Read the model definition and answer for the solid it produces. Units are mm, in the model's axes. A direction names the side the tool comes from. Coordinates: 2 decimals unless noted, no trailing zeros. Write each loop counter-clockwise with the first axis right and the second up, starting at its lowest first coordinate (ties: lowest second). Pieces come first, ordered by that corner, then holes.
1) The part is cut by section A-A (y = 0). Determine the outline of the cut face in (x, z), then the cut area to 4 significant figures.
2) Each of these flat-tipped pins is pushed along its axis until it touches: pin 1 Ø6 at (x, y) = (0, -12.5) entering from +Z; pin 2 Ø7.5 at (x, y) = (0.5, 0.5) entering from -Z; pin 3 Ø7 at (x, z) = (-3.5, 12.5) entering from -Y. Where does it stop, or does it pass through?
3) The part is cut by section C-C (x = 0). Determine the outline of the cut face in (y, z).
4) The part is cut by section D-D (y = 8.25). Determine the outline of the cut face in (x, z).
5) Determine the mould class of faces 1 (the face through (3.5, 0, 7)), 2 (the face through (0, 6, 9)), 3 (the face through (6, 0, 5)), 4 (the face through (10, 0, 0)) for opening direction Y: +Y half, -Y half, draft (parallel to the pull), parting line (faces both ways), or undercut.
6) Find the intervals of material crossed by line 1 (Y direction, x = 0, z = 12); line 2 (X direction, y = 8, z = -0.5); line 3 (Y direction, x = 0, z = -2), in increasing order.
7) The part is cut by section B-B (z = 0). Determine the outline of the cut face in (x, y), then the cut area to 3 significant figures.
8) Which of the six approach directions +Z, -Z, +X, -X, +Y, -Y give full straight-line access (tool end or side, diameter ignored) to faces 5 (the face through (-2, 2, 8.5)), 6 (the face through (-10, -14, 0)), 7 (the face through (-13.274, -11.268, -3.045))?
from build123d import *

# Parameters (mm, degrees)
BOX002_W               = 12.5
BOX002_H               = 5
BOX002_DEPTH           = 10
CYLINDER003_R          = 2
CYLINDER003_DEPTH      = 30
CYLINDER003_ROLL_ANGLE = -90
CYLINDER_R             = 2
CYLINDER_DEPTH         = 30
CYLINDER007_R          = 10
CYLINDER007_DEPTH      = 40
BOX008_W               = 10
BOX008_H               = 2.5
BOX008_DEPTH           = 10
BOX009_W               = 10
BOX009_H               = 2.5
BOX009_DEPTH           = 10
PAD_DEPTH              = 2.5
BOX010_W               = 7
BOX010_H               = 20
BOX010_DEPTH           = 3.5
CYLINDER001_R          = 10
CYLINDER001_DEPTH      = 10
PAD001_DEPTH           = 40
BOX007_W               = 40
BOX007_H               = 30
BOX007_DEPTH           = 10
BOX_W                  = 40
BOX_H                  = 10
BOX_DEPTH              = 12


with BuildPart() as screw_gap:
    # Box002 → Box002 (new body)
    with BuildSketch(Plane(origin=(-20, -2.5, -5), x_dir=(1, 0, 0), z_dir=(0, 0, 1))):
        with Locations((6.25, 2.5)):
            Rectangle(BOX002_W, BOX002_H)
    extrude(amount=BOX002_DEPTH)


with BuildPart() as screw:
    # Cylinder003 → Cylinder003 (new body)
    with BuildSketch(Plane.XY):
        Circle(CYLINDER003_R)
    extrude(amount=CYLINDER003_DEPTH)


with BuildPart() as screw_1:
    # Cylinder003 roll: moved
    add(screw.part.rotate(Axis((0, 0, 0), (1, 0, 0)), CYLINDER003_ROLL_ANGLE))


with BuildPart() as screw_2:
    # Cylinder003 placement: moved
    add(screw_1.part.moved(Location((-15, -15, 0))))


with BuildPart() as rail_screw:
    # Cylinder → Cylinder (new body)
    with BuildSketch(Plane.XY.offset(-5)):
        Circle(CYLINDER_R)
    extrude(amount=CYLINDER_DEPTH)


with BuildPart() as rail:
    # Cylinder007 → Cylinder007 (new body)
    with BuildSketch(Plane(origin=(20, 0, 25), x_dir=(0, 1, 0), z_dir=(-1, 0, 0))):
        Circle(CYLINDER007_R)
    extrude(amount=CYLINDER007_DEPTH)


with BuildPart() as screw_gap001:
    # Box008 → Box008 (new body)
    with BuildSketch(Plane(origin=(-20, 12.5, -5), x_dir=(1, 0, 0), z_dir=(0, 0, 1))):
        with Locations((5, 1.25)):
            Rectangle(BOX008_W, BOX008_H)
    extrude(amount=BOX008_DEPTH)


with BuildPart() as screw_gap002:
    # Box009 → Box009 (new body)
    with BuildSketch(Plane(origin=(-20, -15, -5), x_dir=(1, 0, 0), z_dir=(0, 0, 1))):
        with Locations((5, 1.25)):
            Rectangle(BOX009_W, BOX009_H)
    extrude(amount=BOX009_DEPTH)


with BuildPart() as body:
    # Sketch → Pad (new body)
    with BuildSketch(Plane.XZ):
        Polygon((0, -4.041452), (3.5, -2.020726), (3.5, 2.020726), (0, 4.041452), (-3.5, 2.020726), (-3.5, -2.020726), align=None)
    extrude(amount=-PAD_DEPTH)


with BuildPart() as body_1:
    # Body placement: moved
    add(body.part.moved(Location((-15, -12.5, 0))))


with BuildPart() as cube:
    # Box010 → Box010 (new body)
    with BuildSketch(Plane(origin=(-3.5, -10, 5), x_dir=(1, 0, 0), z_dir=(0, 0, 1))):
        with Locations((3.5, 10)):
            Rectangle(BOX010_W, BOX010_H)
    extrude(amount=BOX010_DEPTH)


with BuildPart() as negative_fusion:
    # Cylinder001 → Cylinder001 (new body)
    with BuildSketch(Plane.XY.offset(-5)):
        Circle(CYLINDER001_R)
    extrude(amount=CYLINDER001_DEPTH)

    # Fusion: union Screw Gap, Screw, Rail Screw, Rail, Screw Gap001, Screw Gap002, Body, Cube
    add(screw_gap.part)
    add(screw_2.part)
    add(rail_screw.part)
    add(rail.part)
    add(screw_gap001.part)
    add(screw_gap002.part)
    add(body_1.part)
    add(cube.part)


with BuildPart() as rail_support_prism:
    # Sketch001 → Pad001 (new body)
    with BuildSketch(Plane.YZ):
        Polygon((5, 0), (10, -5), (-10, -5), (-5, 0), align=None)
    extrude(amount=-PAD001_DEPTH)


with BuildPart() as rail_support_prism_1:
    # Body001 placement: moved
    add(rail_support_prism.part.moved(Location((20, 0, 10))))


with BuildPart() as base_cube:
    # Box007 → Box007 (new body)
    with BuildSketch(Plane(origin=(-20, -15, -5), x_dir=(1, 0, 0), z_dir=(0, 0, 1))):
        with Locations((20, 15)):
            Rectangle(BOX007_W, BOX007_H)
    extrude(amount=BOX007_DEPTH)


with BuildPart() as cut:
    # Box → Box (new body)
    with BuildSketch(Plane(origin=(-20, -5, 5), x_dir=(1, 0, 0), z_dir=(0, 0, 1))):
        with Locations((20, 5)):
            Rectangle(BOX_W, BOX_H)
    extrude(amount=BOX_DEPTH)

    # Fusion002: union Rail Support Prism, Base Cube
    add(rail_support_prism_1.part)
    add(base_cube.part)

    # Cut: cut Negative Fusion
    add(negative_fusion.part, mode=Mode.SUBTRACT)


solid = cut.part
Reported:
1. outline: (-20, 5) - (-3.5, 5) - (-3.5, 8.5) - (-2, 8.5) - (-2, 15) - (-20, 15) - close; (2, 8.5) - (3.5, 8.5) - (3.5, 5) - (10, 5) - (10, -5) - (20, -5) - (20, 15) - (2, 15) - close
1. area: 449.5 mm2
2. pin 1: stops at z = 5
2. pin 2: stops at z = 5
2. pin 3: stops at y = -6
3. outline: (-15, -5) - (-10, -5) - (-10, 5) - (-15, 5) - close; (-6.5, 8.5) - (-2, 8.5) - (-2, 15.2) arc R10 cw to (-5, 16.34) - (-5, 10) - close; (2, 8.5) - (6.5, 8.5) - (5, 10) - (5, 16.34) arc R10 cw to (2, 15.2) - close; (10, -5) - (15, -5) - (15, 5) - (10, 5) - close
4. outline: (-20, -5) - (-5.65, -5) - (-5.65, 5) - (-3.5, 5) - (-3.5, 6.75) - (-20, 6.75) - close; (3.5, 5) - (5.65, 5) - (5.65, -5) - (20, -5) - (20, 6.75) - (3.5, 6.75) - close; hole circle Ø4 at (-15, 0)
5. face 1: draft
5. face 2: +Y half
5. face 3: undercut
5. face 4: undercut
6. line 1: y = -5 to -2, 2 to 5
6. line 2: x = -20 to -16.94, -13.06 to -6, 6 to 20
6. line 3: y = -15 to -10, 10 to 15
7. outline: (-20, -12.5) - (-18.5, -12.5) - (-18.5, -10) - (-17, -10) - (-17, -2.5) - (-20, -2.5) - close; (-20, 2.5) - (-17, 2.5) - (-17, 12.5) - (-20, 12.5) - close; (-13, -10) - (-11.5, -10) - (-11.5, -12.5) - (-10, -12.5) - (-10, -15) - (20, -15) - (20, 15) - (-10, 15) - (-10, 12.5) - (-13, 12.5) - (-13, 2.5) - (-9.68, 2.5) arc R10 cw (long way) to (-9.68, -2.5) - (-13, -2.5) - close
7. area: 698 mm2
8. face 5: -Z, +Y, -Y
8. face 6: +Z, -Z, -X, -Y
8. face 7: -Y
